```python
from build123d import *

# Parameters (mm, degrees)
BOSS_EXTRUDE1_DEPTH = 5
SKETCH2_R           = 1
CUT_EXTRUDE1_DEPTH  = 10


with BuildPart() as part:
    # Sketch1 → Boss-Extrude1 (new, symmetric)
    with BuildSketch(Plane.XY):
        Polygon((-8, 0), (-8, 2), (-10, 2), (-10, 6), (-8, 6), (-8, 8), (-4, 8), (-4, 12), (-2, 12), (-2, 14), (2, 14), (2, 12), (4, 12), (4, 8), (8, 8), (8, 6), (10, 6), (10, 2), (8, 2), (8, 0), align=None)
    extrude(amount=BOSS_EXTRUDE1_DEPTH, both=True)

    # Sketch2 → Cut-Extrude1 (cut)
    with BuildSketch(Plane.XY.offset(5)):
        with Locations((0, 5)):
            Circle(SKETCH2_R)
        with Locations((0, 7.616750923)):
            Circle(SKETCH2_R)
        with Locations((0, 11.414638185)):
            Circle(SKETCH2_R)
        with Locations((-6.151278942, 5)):
            Circle(SKETCH2_R)
        with Locations((5.27484342, 5)):
            Circle(SKETCH2_R)
    extrude(amount=-CUT_EXTRUDE1_DEPTH, mode=Mode.SUBTRACT)


solid = part.part
```
Model file for the job. Use its own axes, mm. A direction names the side the tool comes from. Coordinates: 2 decimals unless noted, no trailing zeros. Order: outer loops, then holes, each group sorted by start corner. A loop starts at its lowest first (then second) coordinate and runs counter-clockwise, first axis right, second up. Notation, with made-up numbers: (-5, -8.75) - (32, -8.75) arc R16 ccw to (32, 4.25) - close; hole circle Ø1 at (1, 31). An arc over 180 degrees is marked (long way). Return JSON: item names as keys, results as strings. Group by question number.
1) Saw through at C-C, the plane x = 4.5. Write the cut outline in (y, z).
2) Probe line 1 (Y direction, x = 0, z = -1); line 2 (Y direction, x = 5.25, z = 4.25); line 3 (Y direction, x = -2.5, z = 3). List the from-to ranges inside material, lowest first. Write a range as from..to.
3) Mould opens along Y. For faces 1 (the flat face through (9, 6, 0)), 2 (the cylindrical face through (0, 6, 0)), 3 (the flat face through (-2, 13, 0)), 4 (the flat face through (0, 0, 0)) say: released by +Y, released by -Y, zero draft, split by the parting line, or undercut.
4) Saw through at B-B, the plane x = 0. Write the cut outline in (y, z), plus the area to 3 significant figures.
5) Tool access for faces 5 (the flat face through (-4, 10, 0)), 6 (the flat face through (-8, 1, 0)), 7 (the flat face through (8, 1, 0)), 8 (the flat face through (8, 7, 0)): list every direction of +Z, -Z, +X, -X, +Y, -Y with a clear straight run to the whole face (end or side of a thin tool).
6) Saw through at A-A, the plane y = 5. Write the cut outline in (x, z), plus the area to 3 significant figures.
7) Saw through at D-D, the plane z = -1.5. Write the cut outline in (x, y), plus the area to 3 significant figures.
8) Flat gauge pins, fed straight in: P1, Ø1.5, axis at x = -4, z = 1, coming from the +Y side; P2, Ø2.5, axis at x = 0, y = 5, coming from the -Z side; P3, Ø4.5, axis at x = 6.5, z = 0, coming from the +Y side; P4, Ø1, axis at y = 9.5, z = -3, coming from the -X side. Where does each tip first touch, or does it go through?
Values found:
{
 "1": {"outline": "(0, -5) - (4.37, -5) - (4.37, 5) - (0, 5) - close; (5.63, -5) - (8, -5) - (8, 5) - (5.63, 5) - close"},
 "2": {"line 1": "y = 0..4, 6..6.62, 8.62..10.41, 12.41..14", "line 2": "y = 0..4, 6..8", "line 3": "y = 0..12"},
 "3": {"face 1": "released by +Y", "face 2": "undercut", "face 3": "zero draft", "face 4": "released by -Y"},
 "4": {"outline": "(0, -5) - (4, -5) - (4, 5) - (0, 5) - close; (6, -5) - (6.62, -5) - (6.62, 5) - (6, 5) - close; (8.62, -5) - (10.41, -5) - (10.41, 5) - (8.62, 5) - close; (12.41, -5) - (14, -5) - (14, 5) - (12.41, 5) - close", "area": "80.0 mm²"},
 "5": {"face 5": "+Z, -Z, -X, +Y", "face 6": "+Z, -Z, -X, -Y", "face 7": "+Z, -Z, +X, -Y", "face 8": "+Z, -Z, +X, +Y"},
 "6": {"outline": "(-10, -5) - (-7.15, -5) - (-7.15, 5) - (-10, 5) - close; (-5.15, -5) - (-1, -5) - (-1, 5) - (-5.15, 5) - close; (1, -5) - (4.27, -5) - (4.27, 5) - (1, 5) - close; (6.27, -5) - (10, -5) - (10, 5) - (6.27, 5) - close", "area": "140 mm²"},
 "7": {"outline": "(-10, 2) - (-8, 2) - (-8, 0) - (8, 0) - (8, 2) - (10, 2) - (10, 6) - (8, 6) - (8, 8) - (4, 8) - (4, 12) - (2, 12) - (2, 14) - (-2, 14) - (-2, 12) - (-4, 12) - (-4, 8) - (-8, 8) - (-8, 6) - (-10, 6) - close; hole circle Ø2 at (-6.15, 5); hole circle Ø2 at (0, 5); hole circle Ø2 at (0, 7.62); hole circle Ø2 at (0, 11.41); hole circle Ø2 at (5.27, 5)", "area": "168 mm²"},
 "8": {"P1": "stops at y = 12", "P2": "stops at z = -5", "P3": "stops at y = 8", "P4": "stops at x = -4"}
}
